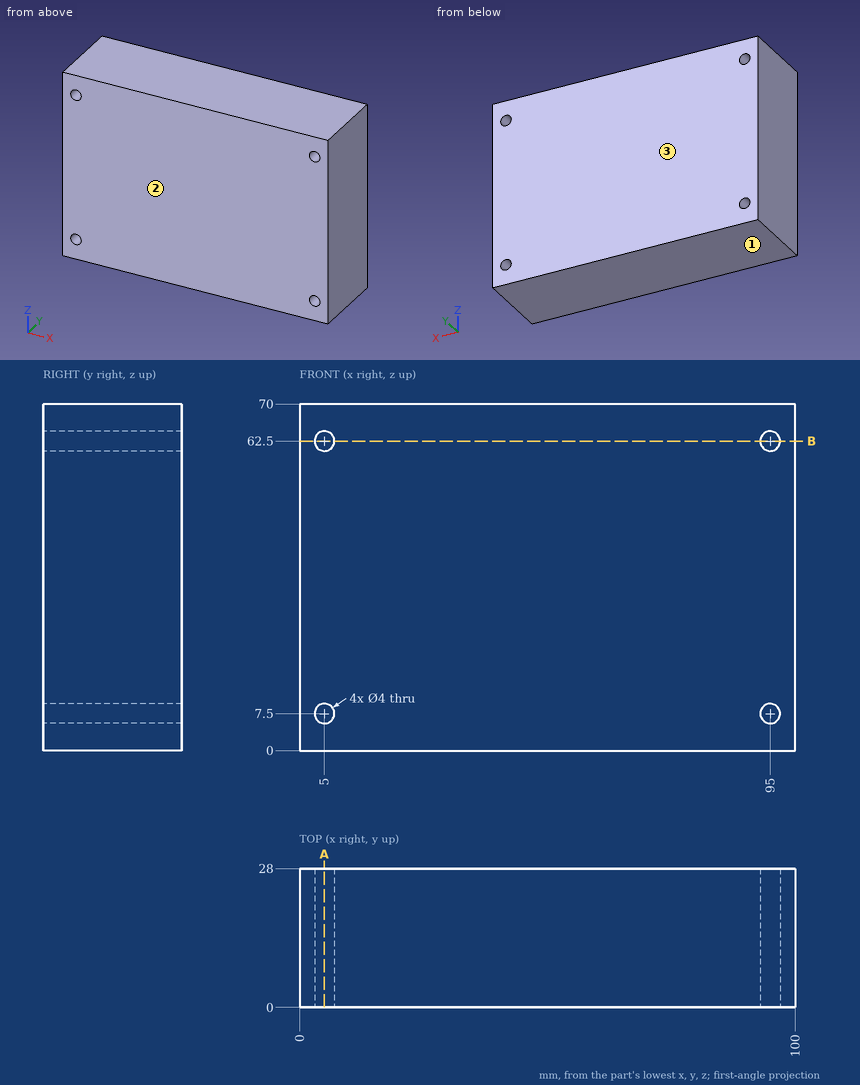
Part print with two shaded views. Sizes in mm from the minimum x, y, z corner. Round coordinates to 2 decimals unless told otherwise and drop trailing zeros. Order: outer loops, then holes, each group sorted by start corner. A loop starts at its lowest first (then second) coordinate and runs counter-clockwise, first axis right, second up. Notation, with made-up numbers: M -12,18 L 25,18 A10 cw 25,23 Z; hole C -28.5,-21.75 d1. An arc over 180 degrees is marked long. Use CSV: the item, a comma, the result in double quotes. Start each with the question number.
(1) Mould opens along Y. For the marked faces 1, 2 and 3 say: +Y half, -Y half, draft (parallel to the pull), parting line (faces both ways), or undercut.
(2) Drill centre lines: probe 1 along Z at (x, y) = (95, 7.75); probe 2 along Z at (x, y) = (94.5, 21.75). Where is each one in solid material? Low to high.
(3) Cut at B-B on z = 62.5. List the corners of the cut face in (x, y), then the cut area to 3 significant figures.
(4) Flat gauge pin, fed straight in: P1, Ø3.5, axis at x = 95, z = 62.5, coming from the -Y side. Where does the tip first touch, or does it go through?
(5) Cut at A-A on x = 5. List the corners of the cut face in (y, z), then the cut area to 3 significant figures.
Findings:
1,face 1,"draft"
1,face 2,"-Y half"
1,face 3,"+Y half"
2,probe 1,"z = 0 to 5.5, 9.5 to 60.5, 64.5 to 70"
2,probe 2,"z = 0 to 5.56, 9.44 to 60.56, 64.44 to 70"
3,outline,"M 0,0 L 3,0 L 3,28 L 0,28 Z; M 7,0 L 93,0 L 93,28 L 7,28 Z; M 97,0 L 100,0 L 100,28 L 97,28 Z"
3,area,"2,580 mm^2"
4,P1,"passes through"
5,outline,"M 0,0 L 28,0 L 28,5.5 L 0,5.5 Z; M 0,9.5 L 28,9.5 L 28,60.5 L 0,60.5 Z; M 0,64.5 L 28,64.5 L 28,70 L 0,70 Z"
5,area,"1,740 mm^2"
